```python
from build123d import *

# Parameters (mm, degrees)
F0_W         = 198.7862437963
F0_H         = 84.2363908887
F1_DEPTH     = 87.63
F2_DEPTH     = 30.226
F3_DEPTH     = 38.1
F4_DEPTH     = 36.068
F5_W         = 118.6288297176
F5_H         = 62.8803037107
F6_DEPTH     = 119.38
F7_W         = 114.9956956506
F7_H         = 23.0015479028
F8_DEPTH     = 114.3
F9_DEPTH     = 216.916
F10_DEPTH    = 97.282
F11_W        = 95.1088294387
F11_H        = 86.9466327131
F14_DEPTH    = 121.666
F12_W        = 30.4002016783
F12_H        = 84.9931621924
F15_DEPTH    = 121.666
F13_W        = 29.6071916819
F13_H        = 84.3174913898
F16_DEPTH    = 121.666
F18_W        = 155.8008268476
F18_H        = 43.2829973288
F19_DEPTH    = 121.666
F17_W        = 126.6549825668
F17_H        = 42.8492124192
F20_DEPTH    = 121.666
F21_T1_DEPTH = 680.2142882536


# Not quite as in the source:
# - a fillet or chamfer that OpenCascade refuses, or shapes differently, is made with other operations: its cross-section is extruded or revolved along the edge and cut away or added


with BuildPart() as f1:
    # F0 (on Top) → F1 (new body)
    with BuildSketch(Plane.XY):
        Rectangle(F0_W, F0_H)
    extrude(amount=F1_DEPTH)

    # F2 (add): a face of the model
    f2_faces = [f1.faces().sort_by_distance(p)[0] for p in [
        (0, -42.1181954443, 43.815),
    ]]
    extrude(f2_faces, amount=F2_DEPTH)

    # F3 (add): a face of the model
    f3_faces = [f1.faces().sort_by_distance(p)[0] for p in [
        (0, -15.113, 0),
    ]]
    extrude(f3_faces, amount=F3_DEPTH)

    # F4 (add): a face of the model
    f4_faces = [f1.faces().sort_by_distance(p)[0] for p in [
        (0, -72.3441954443, 24.765),
    ]]
    extrude(f4_faces, amount=F4_DEPTH)

    # F5 (on face) → F6 (cut)
    with BuildSketch(Plane.XY.offset(87.63)):
        with Locations((31.7698940635, -71.2347794324)):
            Rectangle(F5_W, F5_H)
    extrude(amount=-F6_DEPTH, mode=Mode.SUBTRACT)

    # F7 (on face) → F8 (cut)
    with BuildSketch(Plane.XY.offset(87.63)):
        with Locations((32.1380235255, -23.2001785189)):
            Rectangle(F7_W, F7_H)
    extrude(amount=-F8_DEPTH, mode=Mode.SUBTRACT)

    # F9 (add): a face of the model
    f9_faces = [f1.faces().sort_by_distance(p)[0] for p in [
        (-99.3931218982, -33.147, 24.765),
    ]]
    extrude(f9_faces, amount=F9_DEPTH)

    # F10 (cut): a face of the model
    f10_faces = [f1.faces().sort_by_distance(p)[0] for p in [
        (-316.3091218982, -33.147, 24.765),
    ]]
    extrude(f10_faces, amount=-F10_DEPTH, mode=Mode.SUBTRACT)

    # F11 (on face) → F14 (cut)
    with BuildSketch(Plane.XY.offset(87.63)):
        with Locations((-83.8001854718, -56.8147618324)):
            Rectangle(F11_W, F11_H)
    extrude(amount=-F14_DEPTH, mode=Mode.SUBTRACT)

    # F12 (on face) → F15 (cut)
    with BuildSketch(Plane.XY.offset(87.63)):
        with Locations((-155.1787778735, -56.0720595531)):
            Rectangle(F12_W, F12_H)
    extrude(amount=-F15_DEPTH, mode=Mode.SUBTRACT)

    # F13 (on face) → F16 (cut)
    with BuildSketch(Plane.XY.offset(87.63)):
        with Locations((-193.8888058066, -55.9172849171)):
            Rectangle(F13_W, F13_H)
    extrude(amount=-F16_DEPTH, mode=Mode.SUBTRACT)

    # F18 (on face) → F19 (cut)
    with BuildSketch(Plane.XY.offset(87.63)):
        with Locations((9.4717927277, 15.8045829739)):
            Rectangle(F18_W, F18_H)
    extrude(amount=-F19_DEPTH, mode=Mode.SUBTRACT)

    # F17 (on face) → F20 (cut)
    with BuildSketch(Plane.XY.offset(87.63)):
        with Locations((-145.3649103642, 15.8879833762)):
            Rectangle(F17_W, F17_H)
    extrude(amount=-F20_DEPTH, mode=Mode.SUBTRACT)

    # F21: fillet of radius 72.3588088914 on 1 edges, made by hand

    # F21_s2 → F21_t1 (cut)
    with BuildSketch(Plane.YZ.offset(-399.9241441268)):
        with BuildLine():
            ThreePointArc((42.1181954443, 15.2711911086), (20.9247909986, 66.4365955543), (-30.2406134471, 87.63))
            Line((-30.2406134471, 87.63), (42.1181954443, 87.63))
            Line((42.1181954443, 87.63), (42.1181954443, 15.2711911086))
        make_face()
    extrude(amount=F21_T1_DEPTH, mode=Mode.SUBTRACT)


solid = f1.part
```
Could you check a few things on this model? Use its own coordinates, in mm. A direction names the side the tool comes from. Give positions to 0.01 mm unless a question says otherwise; leave off trailing zeros. Loops run counter-clockwise (first coordinate to the right, second up) from the corner with the lowest first, then second, coordinate; pieces in that order, holes last. Notation, with made-up numbers: (35, 28) -> (92, 28) arc R20 ccw to (92, 53) -> close; hole circle Ø1 at (87.5, 19.25). An arc over 180 degrees is marked (long way). Put each result on its own line as item: value.
(1) Imagine slicing it at A-A on z = -21. State how many separate pieces and enclosed holes the cut face has, plus the area to 3 significant figures.
Computed:
separate pieces: 1
enclosed holes: 7
area: 12,300 mm^2
(2) For faces 1 (the face through (-68.429, 16, 25)), 2 (the face through (-36.97, 38.53, 37.78)), which set-ups out of +Z, -Z, +X, -X, +Y, -Y let a thin tool reach every point of the face, with its end or its side?
Computed:
face 1: +Z
face 2: +Z, +X, -X, +Y
(3) Please list where these lines run through material, in increasing order: probe 1 along X at (y, z) = (-51.5, 76.5); probe 2 along Y at (x, z) = (-50, -8); probe 3 along X at (y, z) = (-23, 5). Write a range as [from, to].
Computed:
probe 1: [-219.03, -208.69], [-179.09, -170.38], [-139.98, -131.35], [-36.25, -27.54], [91.08, 99.39]
probe 2: [-108.41, -100.29], [-13.34, -5.84], [37.45, 42.12]
probe 3: [-219.03, -208.69], [-179.09, -170.38], [-139.98, -131.35], [-36.25, -25.36], [89.64, 99.39]
(4) Thinking about a two-plate mould opening in X: for faces 3 (the face through (89.636, -23, 31)), 4 (the face through (-59, -101, 87.63)), which applies, pulls with the +X half, pulls with the -X half, needs draft (parallel to the pull), parting line crosses it, or undercut?
Computed:
face 3: undercut
face 4: needs draft
(5) Imagine slicing it at C-C on y = -87.5. Write out the boundary of the cut face in (x, z).
Computed:
outline: (-219.03, -38.1) -> (99.39, -38.1) -> (99.39, 87.63) -> (91.08, 87.63) -> (91.08, -31.75) -> (-27.54, -31.75) -> (-27.54, 87.63) -> (-36.25, 87.63) -> (-36.25, -34.04) -> (-131.35, -34.04) -> (-131.35, 87.63) -> (-139.98, 87.63) -> (-139.98, -34.04) -> (-170.38, -34.04) -> (-170.38, 87.63) -> (-179.09, 87.63) -> (-179.09, -34.04) -> (-208.69, -34.04) -> (-208.69, 87.63) -> (-219.03, 87.63) -> close
(6) Imagine slicing it at B-B on x = -176. Write out the boundary of the cut face in (y, z), plus the area to 3 significant figures.
Computed:
outline: (-108.41, -38.1) -> (42.12, -38.1) -> (42.12, 15.27) arc R72.36 ccw to (37.31, 41.2) -> (37.31, -34.04) -> (-5.54, -34.04) -> (-5.54, 83.28) arc R72.36 ccw to (-30.24, 87.63) -> (-108.41, 87.63) -> close
area: 13,400 mm^2
(7) I'm going to push flat-ended pins straight in: pin 1 Ø4 at (x, z) = (7.5, 37) entering from +Y; pin 2 Ø11.5 at (x, y) = (37, -18) entering from +Z; pin 3 Ø10 at (x, y) = (-86.5, 7) entering from +Z. Where does each tip first touch, or does it pass through?
Computed:
pin 1: y = 39.38
pin 2: z = -26.67
pin 3: z = 78.61
